Part model, mm, in its own coordinate system. A direction names the side the tool comes from. Round coordinates to 2 decimals unless told otherwise and drop trailing zeros. Loops run counter-clockwise (first coordinate to the right, second up) from the corner with the lowest first, then second, coordinate; pieces in that order, holes last.
1) Band-saw the part on B-B, the plane y = -243. Write the cut outline in (x, z), then the cut area to 3 significant figures.
2) Band-saw the part on A-A, the plane x = 0. Write the cut outline in (y, z), then the cut area to 3 significant figures.
3) 3-axis set-ups, long thin cutter, end or side, ignore diameter. For faces 1 (the flat face through (0, 0, 0)), 2 (the flat face through (1, -116, -0.5)): which of +Z, -Z, +X, -X, +Y, -Y reach the whole face in a straight line?
4) Band-saw the part on C-C, the plane z = -9.75. Write the cut outline in (x, y).
5) Mould opens along X. For faces 3 (the flat face through (1, -188, -0.5)), 4 (the flat face through (0, -310, 0)), 5 (the cylindrical face through (-3.03, -152.83, -13.67)) say: +X half, -X half, draft (parallel to the pull), parting line (faces both ways), or undercut.
6) Probe line 1 (Y direction, x = 0.25, z = 10); line 2 (Y direction, x = 7.5, z = 7.5); line 3 (X direction, y = -249, z = 1.25). List the from-to ranges inside material, lowest first.
7) Band-saw the part on D-D, the plane y = -144. Write the cut outline in (x, z), then the cut area to 3 significant figures.
8) Drop flat-ended pins along their axis: P1, Ø7, axis at x = 3, z = 8, coming from the +Y side; P2, Ø6.5, axis at y = -186.5, z = 7, coming from the +X side; P3, Ø4, axis at x = 2, y = -199.5, coming from the +Z side; P4, Ø3.5, axis at y = -29.5, z = 4.5, coming from the -X side. Give the stop position or say it passes through.
from build123d import *

# Parameters (mm, degrees)
F0_R     = 14
F1_DEPTH = 310
F3_W     = 14.182319
F3_H     = 39.444565
F3_W_2   = 13.73912
F3_H_2   = 49.19491
F3_W_3   = 13.295921
F3_H_3   = 46.978921
F3_W_4   = 17.2847
F3_H_4   = 54.513276
F4_DEPTH = 15


with BuildPart() as f1:
    # F0 (on Front) → F1 (new body)
    with BuildSketch(Plane.XZ):
        Circle(F0_R)
    extrude(amount=F1_DEPTH)

    # F3 (on offset) → F4 (cut)
    with BuildSketch(Plane.XY.offset(14.5)):
        with Locations((1.216165, -30.746452)):
            Rectangle(F3_W, F3_H)
        with Locations((1.437765, -116.283547)):
            Rectangle(F3_W_2, F3_H_2)
        with Locations((0.772966, -187.859922)):
            Rectangle(F3_W_3, F3_H_3)
        with Locations((1.880962, -260.32269)):
            Rectangle(F3_W_4, F3_H_4)
    extrude(amount=-F4_DEPTH, mode=Mode.SUBTRACT)


solid = f1.part
Reported:
1. outline: (-6.76, -0.5) - (-6.76, 12.26) arc R14 ccw (long way) to (10.52, 9.23) - (10.52, -0.5) - close
1. area: 384 mm2
2. outline: (-310, -14) - (0, -14) - (0, 14) - (-11.02, 14) - (-11.02, -0.5) - (-50.47, -0.5) - (-50.47, 14) - (-91.69, 14) - (-91.69, -0.5) - (-140.88, -0.5) - (-140.88, 14) - (-164.37, 14) - (-164.37, -0.5) - (-211.35, -0.5) - (-211.35, 14) - (-233.07, 14) - (-233.07, -0.5) - (-287.58, -0.5) - (-287.58, 14) - (-310, 14) - close
2. area: 5,920 mm2
3. face 1: +Z, -Z, +X, -X, +Y
3. face 2: +Z
4. outline: (-10.05, -310) - (10.05, -310) - (10.05, 0) - (-10.05, 0) - close
5. face 3: undercut
5. face 4: draft
5. face 5: parting line
6. line 1: y = -310 to -287.58, -233.07 to -211.35, -164.37 to -140.88, -91.69 to -50.47, -11.02 to 0
6. line 2: y = -310 to -287.58, -233.07 to -140.88, -91.69 to -50.47, -11.02 to 0
6. line 3: x = -13.94 to -6.76, 10.52 to 13.94
7. outline: circle Ø28 at (0, 0)
7. area: 616 mm2
8. P1: stops at y = 0
8. P2: stops at x = 13.49
8. P3: stops at z = -0.5
8. P4: stops at x = -13.73
